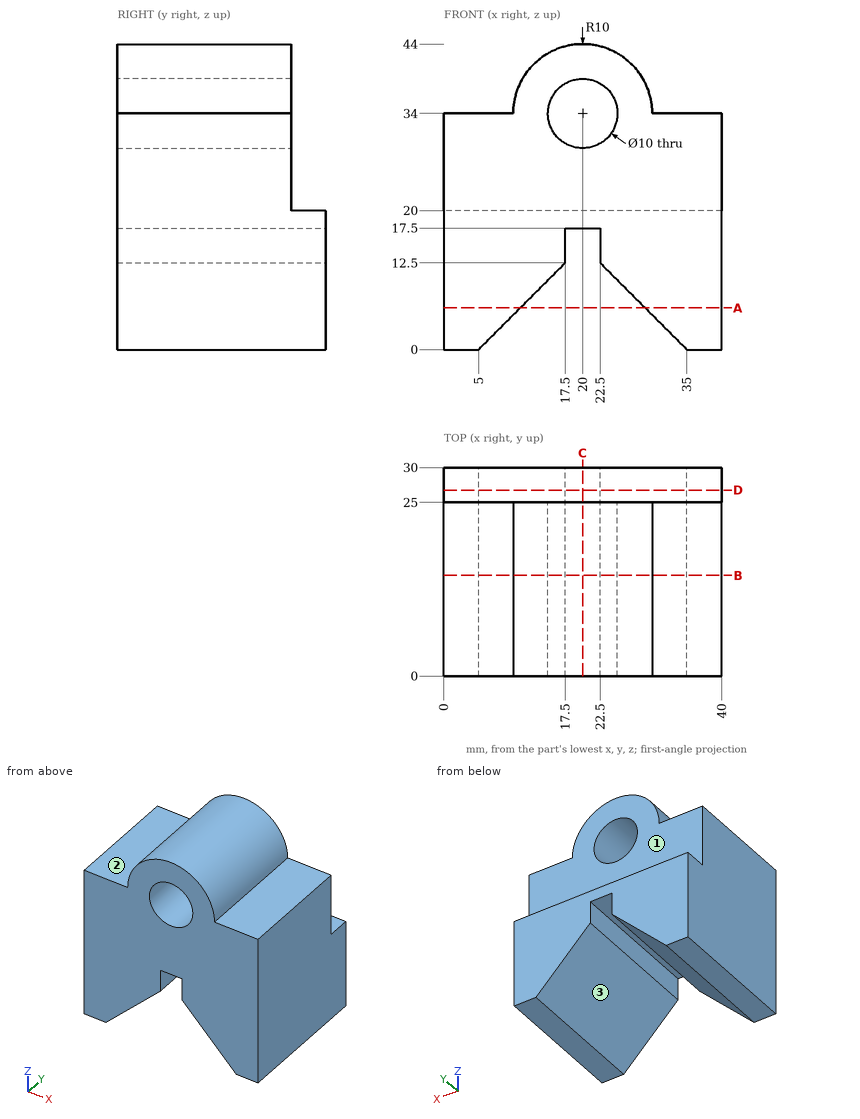
Part print with two shaded views. Sizes in mm from the minimum x, y, z corner. A direction names the side the tool comes from. Coordinates: 2 decimals unless noted, no trailing zeros. Write each loop counter-clockwise with the first axis right and the second up, starting at its lowest first coordinate (ties: lowest second). Pieces come first, ordered by that corner, then holes. Notation, with made-up numbers: (25.25, 41.25) - (30.25, 41.25) arc R27 cw to (30.25, 69.25) - close; hole circle Ø1 at (62, 66). An arc over 180 degrees is marked (long way). Use a Markdown table: item, result. Add a question column.
Item 1: Band-saw the part on D-D, the plane y = 26.75. Write the cut outline in (x, z).
Item 2: Drop flat-ended pins along their axis: pin 1 (1.5 mm diameter, centred on x = 11, y = 26, fed in from -Z); pin 2 (2.5 mm diameter, centred on x = 19, y = 20.5, fed in from -Z); pin 3 (8 mm diameter, centred on x = 14, y = 20.5, fed in from +Z). Give the stop position or say it passes through.
Item 3: Band-saw the part on C-C, the plane x = 20. Write the cut outline in (y, z), and give its area (3 significant figures).
Item 4: Band-saw the part on A-A, the plane z = 6. Write the cut outline in (x, y).
Item 5: Band-saw the part on B-B, the plane y = 14.5. Write the cut outline in (x, z).
Item 6: Drill centre lines: line 1 along X through (y, z) = (2, 14.5); line 2 along X through (y, z) = (26.5, 5.5); line 3 along Z through (x, y) = (24.5, 24). Where is each one in solid material? Low to high.
Item 7: 3-axis set-ups, long thin cutter, end or side, ignore diameter. For the marked faces 1, 2 and 3: which of +Z, -Z, +X, -X, +Y, -Y reach the whole face in a straight line?
A:
| question | item | result |
|---|---|---|
| 1 | outline | (0, 0) - (5, 0) - (17.5, 12.5) - (17.5, 17.5) - (22.5, 17.5) - (22.5, 12.5) - (35, 0) - (40, 0) - (40, 20) - (0, 20) - close |
| 2 | pin 1 | stops at z = 5.25 |
| 2 | pin 2 | stops at z = 17.5 |
| 2 | pin 3 | stops at z = 43.8 |
| 3 | outline | (0, 17.5) - (30, 17.5) - (30, 20) - (25, 20) - (25, 29) - (0, 29) - close; (0, 39) - (25, 39) - (25, 44) - (0, 44) - close |
| 3 | area | 425 mm² |
| 4 | outline | (0, 0) - (11, 0) - (11, 30) - (0, 30) - close; (29, 0) - (40, 0) - (40, 30) - (29, 30) - close |
| 5 | outline | (0, 0) - (5, 0) - (17.5, 12.5) - (17.5, 17.5) - (22.5, 17.5) - (22.5, 12.5) - (35, 0) - (40, 0) - (40, 34) - (30, 34) arc R10 ccw to (10, 34) - (0, 34) - close; hole circle Ø10 at (20, 34) |
| 6 | line 1 | x = 0 to 17.5, 22.5 to 40 |
| 6 | line 2 | x = 0 to 10.5, 29.5 to 40 |
| 6 | line 3 | z = 10.5 to 31.82, 36.18 to 42.93 |
| 7 | face 1 | +Z, +X, -X, +Y |
| 7 | face 2 | +Z, -X, +Y, -Y |
| 7 | face 3 | -Z, +Y, -Y |
